Verification items for this drawing (mm, ordinates from the low corner). Coordinates: 2 decimals unless noted, no trailing zeros. Order: outer loops, then holes, each group sorted by start corner. A loop starts at its lowest first (then second) coordinate and runs counter-clockwise, first axis right, second up. Notation, with made-up numbers: M -21,88 L -7,88 A16 cw -7,119 Z; hole C -12,21 d4. An arc over 180 degrees is marked long. Answer as a JSON object with one key per item and string values. Group by question number.
(1) Gauge pin test, flat end, axial feed: pin 1 Ø1.5 at (x, z) = (56, 115.5) entering from -Y. Record the tip position at first contact, or that the pin passes through.
(2) Cross-section at B-B (z = 13). Enter the section's corners in (x, y).
(3) Material ranges on line 1 (Z direction, x = 57.5, y = 3.75); line 2 (X direction, y = 4, z = 54); line 3 (Y direction, x = 27, z = 67), recorded low to high.
(4) Mould release check, pull along Z, two halves, no side actions. Record for the marked faces 1 and 2: released by +Z, released by -Z, zero draft, split by the parting line, or undercut.
(5) Cross-section at A-A (y = 1.5). Enter the section's corners in (x, z), plus the area to 3 significant figures.
(6) Cross-section at C-C (x = 58.5). Enter the section's corners in (y, z), plus the area to 3 significant figures.
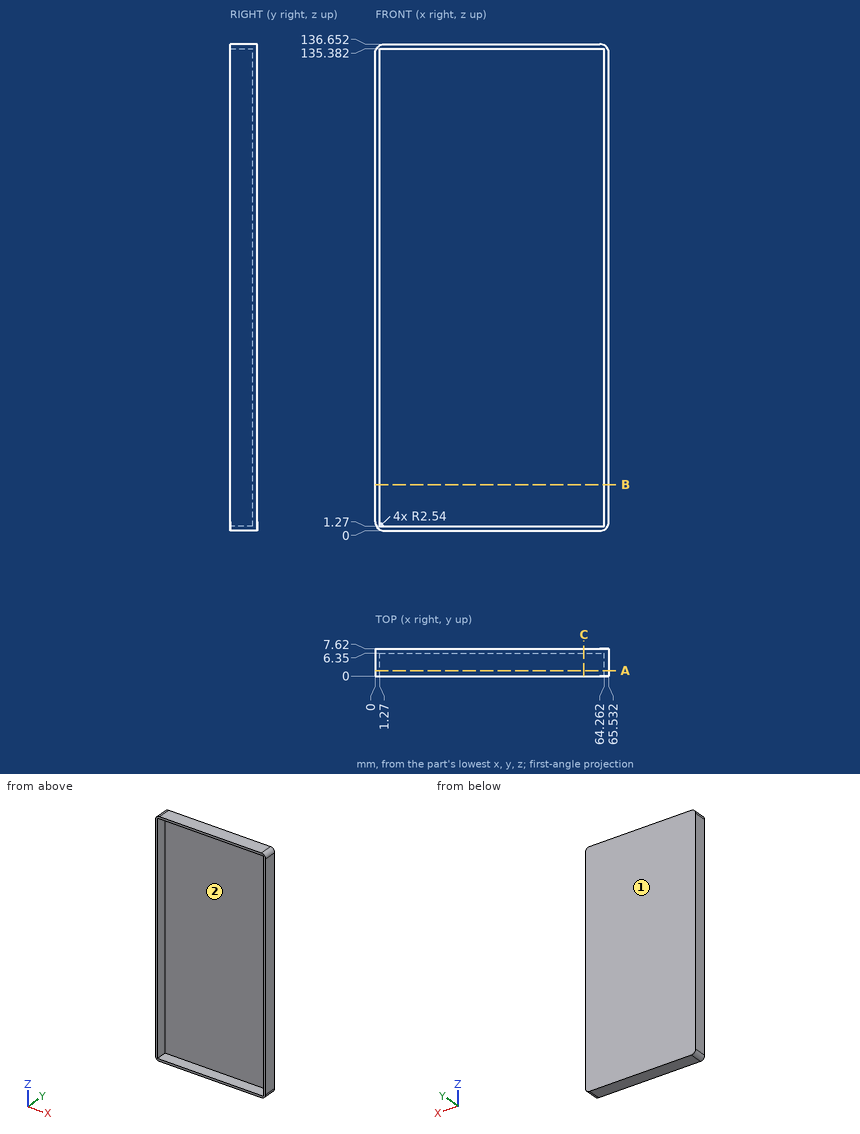
Taken from the geometry:
{
 "1": {"pin 1": "stops at y = 6.35"},
 "2": {"outline": "M 0,0 L 1.27,0 L 1.27,6.35 L 64.26,6.35 L 64.26,0 L 65.53,0 L 65.53,7.62 L 0,7.62 Z"},
 "3": {"line 1": "z = 0 to 1.27, 135.38 to 136.65", "line 2": "x = 0 to 1.27, 64.26 to 65.53", "line 3": "y = 6.35 to 7.62"},
 "4": {"face 1": "zero draft", "face 2": "undercut"},
 "5": {"outline": "M 0,2.54 A2.54 ccw 2.54,0 L 62.99,0 A2.54 ccw 65.53,2.54 L 65.53,134.11 A2.54 ccw 62.99,136.65 L 2.54,136.65 A2.54 ccw 0,134.11 Z; hole M 1.27,1.27 L 64.26,1.27 L 64.26,135.38 L 1.27,135.38 Z", "area": "502 mm²"},
 "6": {"outline": "M 0,0 L 7.62,0 L 7.62,136.65 L 0,136.65 L 0,135.38 L 6.35,135.38 L 6.35,1.27 L 0,1.27 Z", "area": "190 mm²"}
}
